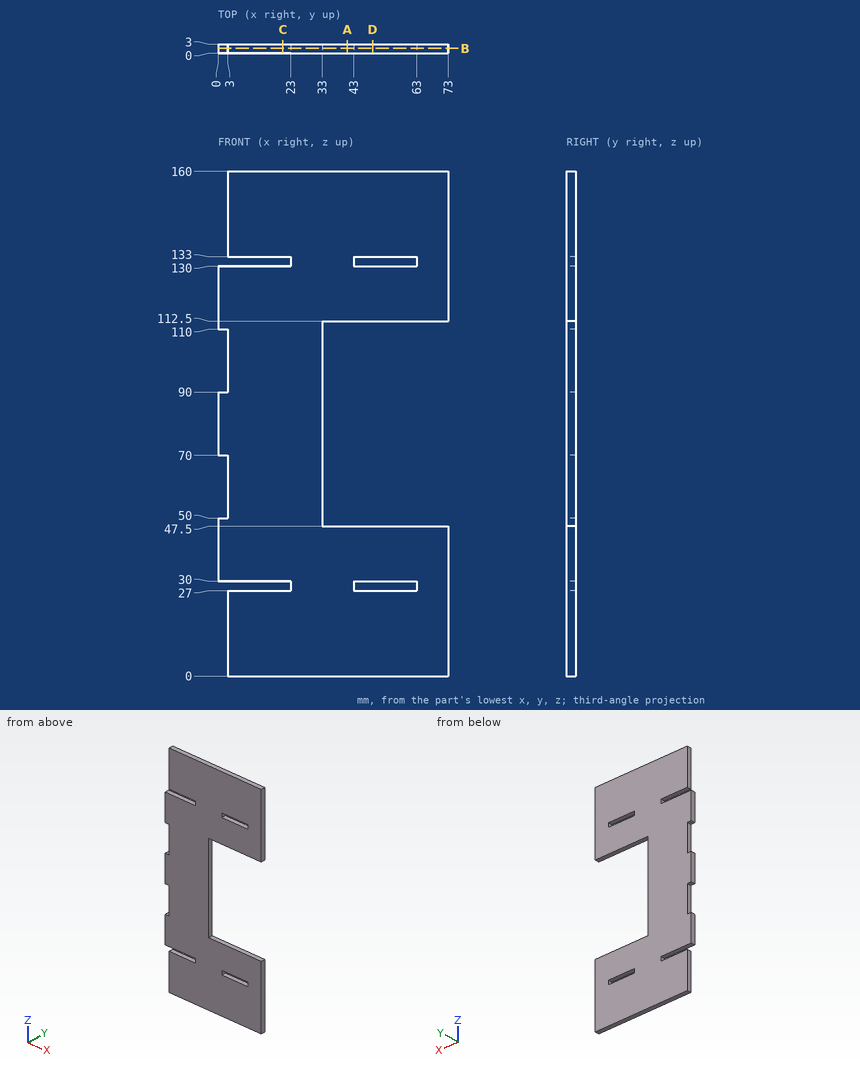
For this review, use the dimensioned drawing (mm, ordinates from the lowest corner) and the shaded views. Coordinates: 2 decimals unless noted, no trailing zeros. Order: outer loops, then holes, each group sorted by start corner. A loop starts at its lowest first (then second) coordinate and runs counter-clockwise, first axis right, second up. Notation, with made-up numbers: (-12, 66.25) - (-2, 66.25) arc R16 ccw to (-2, 82.25) - close; hole circle Ø5 at (-5.5, -17.5). An arc over 180 degrees is marked (long way). Answer as a JSON object with one key per item and string values. Group by question number.
1. Clearance check with flat-ended pins moving along their axes: P1, Ø1.5, axis at x = 55.5, y = 1, coming from the -Z side; P2, Ø1.5, axis at y = 1.5, z = 147.5, coming from the -X side; P3, Ø0.9, axis at x = 1, y = 1.5, coming from the -Z side; P4, Ø0.9, axis at y = 2, z = 88.5, coming from the +X side. State where each tip first meets the part, or that it passes through.
2. We need section B-B on y = 1.6. Give the number of separate pieces and of enclosed holes in the cut face, then the cut area to 3 significant figures.
3. For probe 1 along Z at (x, y) = (53.5, 0.75); probe 2 along Z at (x, y) = (20, 0.85); probe 3 along Z at (x, y) = (40, 1.9), list the stretches that pass through material, from the lowest coordinate up.
4. We need section C-C on x = 20.5. State the section outline as (y, z) points, then the cut area to 3 significant figures.
5. We need section A-A on x = 41. State the section outline as (y, z) points, then the cut area to 3 significant figures.
6. We need section D-D on x = 49. State the section outline as (y, z) points, then the cut area to 3 significant figures.
Final values:
{
 "1": {"P1": "z = 0", "P2": "x = 3", "P3": "z = 30", "P4": "x = 33"},
 "2": {"separate pieces": "1", "enclosed holes": "2", "area": "8,540 mm²"},
 "3": {"probe 1": "0 to 27, 30 to 47.5, 112.5 to 130, 133 to 160", "probe 2": "0 to 27, 30 to 130, 133 to 160", "probe 3": "0 to 47.5, 112.5 to 160"},
 "4": {"outline": "(0, 0) - (3, 0) - (3, 27) - (0, 27) - close; (0, 30) - (3, 30) - (3, 130) - (0, 130) - close; (0, 133) - (3, 133) - (3, 160) - (0, 160) - close", "area": "462 mm²"},
 "5": {"outline": "(0, 0) - (3, 0) - (3, 47.5) - (0, 47.5) - close; (0, 112.5) - (3, 112.5) - (3, 160) - (0, 160) - close", "area": "285 mm²"},
 "6": {"outline": "(0, 0) - (3, 0) - (3, 27) - (0, 27) - close; (0, 30) - (3, 30) - (3, 47.5) - (0, 47.5) - close; (0, 112.5) - (3, 112.5) - (3, 130) - (0, 130) - close; (0, 133) - (3, 133) - (3, 160) - (0, 160) - close", "area": "267 mm²"}
}
